from build123d import *

# Parameters (mm, degrees)
SKETCH_3_W          = 220
SKETCH_3_H          = 130
EXTRUDE_1_DEPTH     = 5
CUT_EXTRUDE_1_DEPTH = 6
SKETCH_3_4_W        = 220
SKETCH_3_4_H        = 13
EXTRUDE_2_DEPTH     = 15


with BuildPart() as part:
    # Sketch 3 → Extrude 1 (new body)
    with BuildSketch(Plane.XY):
        Rectangle(SKETCH_3_W, SKETCH_3_H)
    extrude(amount=EXTRUDE_1_DEPTH)

    # Sketch 3_3 → Cut-Extrude 1 (cut, through all)
    with BuildSketch(Plane.XY):
        Polygon((75.116731493, -11.546415335), (85.057854749, -5.672115229), (84.941123256, 5.874300106), (74.883268507, 11.546415335), (64.942145251, 5.672115229), (65.058876744, -5.874300106), align=None)
        Polygon((50.116731493, -11.546415335), (60.057854749, -5.672115229), (59.941123256, 5.874300106), (49.883268507, 11.546415335), (39.942145251, 5.672115229), (40.058876744, -5.874300106), align=None)
        Polygon((50.116731493, -41.546415335), (60.057854749, -35.672115229), (59.941123256, -24.125699894), (49.883268507, -18.453584665), (39.942145251, -24.327884771), (40.058876744, -35.874300106), align=None)
        Polygon((25.116731493, -41.546415335), (35.057854749, -35.672115229), (34.941123256, -24.125699894), (24.883268507, -18.453584665), (14.942145251, -24.327884771), (15.058876744, -35.874300106), align=None)
        Polygon((25.116731493, -11.546415335), (35.057854749, -5.672115229), (34.941123256, 5.874300106), (24.883268507, 11.546415335), (14.942145251, 5.672115229), (15.058876744, -5.874300106), align=None)
        Polygon((0.116731493, -41.546415335), (10.057854749, -35.672115229), (9.941123256, -24.125699894), (-0.116731493, -18.453584665), (-10.057854749, -24.327884771), (-9.941123256, -35.874300106), align=None)
        Polygon((-24.884546065, -41.546415335), (-14.943422809, -35.672115229), (-15.060154302, -24.125699894), (-25.118009051, -18.453584665), (-35.059132307, -24.327884771), (-34.942400814, -35.874300106), align=None)
        Polygon((-24.884546065, -11.546415335), (-14.943422809, -5.672115229), (-15.060154302, 5.874300106), (-25.118009051, 11.546415335), (-35.059132307, 5.672115229), (-34.942400814, -5.874300106), align=None)
        Polygon((0.116731493, -11.546415335), (10.057854749, -5.672115229), (9.941123256, 5.874300106), (-0.116731493, 11.546415335), (-10.057854749, 5.672115229), (-9.941123256, -5.874300106), align=None)
        Polygon((-49.885823623, -41.546415335), (-39.944700367, -35.672115229), (-40.06143186, -24.125699894), (-50.119286609, -18.453584665), (-60.060409866, -24.327884771), (-59.943678372, -35.874300106), align=None)
        Polygon((-49.885823623, -11.546415335), (-39.944700367, -5.672115229), (-40.06143186, 5.874300106), (-50.119286609, 11.546415335), (-60.060409866, 5.672115229), (-59.943678372, -5.874300106), align=None)
        Polygon((-74.887101181, -41.546415335), (-64.945977925, -35.672115229), (-65.062709418, -24.125699894), (-75.120564167, -18.453584665), (-85.061687424, -24.327884771), (-84.944955931, -35.874300106), align=None)
        Polygon((-74.887101181, 18.453584665), (-64.945977925, 24.327884771), (-65.062709418, 35.874300106), (-75.120564167, 41.546415335), (-85.061687424, 35.672115229), (-84.944955931, 24.125699894), align=None)
        Polygon((-49.885823623, 18.453584665), (-39.944700367, 24.327884771), (-40.06143186, 35.874300106), (-50.119286609, 41.546415335), (-60.060409866, 35.672115229), (-59.943678372, 24.125699894), align=None)
        Polygon((-24.884546065, 18.453584665), (-14.943422809, 24.327884771), (-15.060154302, 35.874300106), (-25.118009051, 41.546415335), (-35.059132307, 35.672115229), (-34.942400814, 24.125699894), align=None)
        Polygon((0.116731493, 18.453584665), (10.057854749, 24.327884771), (9.941123256, 35.874300106), (-0.116731493, 41.546415335), (-10.057854749, 35.672115229), (-9.941123256, 24.125699894), align=None)
        Polygon((25.116731493, 18.453584665), (35.057854749, 24.327884771), (34.941123256, 35.874300106), (24.883268507, 41.546415335), (14.942145251, 35.672115229), (15.058876744, 24.125699894), align=None)
        Polygon((50.116731493, 18.453584665), (60.057854749, 24.327884771), (59.941123256, 35.874300106), (49.883268507, 41.546415335), (39.942145251, 35.672115229), (40.058876744, 24.125699894), align=None)
        Polygon((75.116731493, 18.453584665), (85.057854749, 24.327884771), (84.941123256, 35.874300106), (74.883268507, 41.546415335), (64.942145251, 35.672115229), (65.058876744, 24.125699894), align=None)
        Polygon((85.057854749, -35.672115229), (84.941123256, -24.125699894), (74.883268507, -18.453584665), (64.942145251, -24.327884771), (65.058876744, -35.874300106), (75.116731493, -41.546415335), align=None)
        Polygon((-74.887101181, -11.546415335), (-64.945977925, -5.672115229), (-65.062709418, 5.874300106), (-75.120564167, 11.546415335), (-85.061687424, 5.672115229), (-84.944955931, -5.874300106), align=None)
    extrude(amount=CUT_EXTRUDE_1_DEPTH, mode=Mode.SUBTRACT)

    # Sketch 3_4 → Extrude 2 (add)
    with BuildSketch(Plane.XY):
        with Locations((0, 58.5)):
            Rectangle(SKETCH_3_4_W, SKETCH_3_4_H)
        with Locations((0, -58.5)):
            Rectangle(SKETCH_3_4_W, SKETCH_3_4_H)
    extrude(amount=EXTRUDE_2_DEPTH)


solid = part.part
Build history of the part. All positions in model axes, mm. Coordinates: 2 decimals unless noted, no trailing zeros. Write each loop counter-clockwise with the first axis right and the second up, starting at its lowest first coordinate (ties: lowest second). Pieces come first, ordered by that corner, then holes.
(1) Drill centre lines: line 1 (Y direction, x = 31, z = 13.25); line 2 (Y direction, x = 8, z = 1.5); line 3 (Z direction, x = -15, y = 22.5). Where is each one in solid material? Low to high.
(2) Cut at D-D on x = 19. List the corners of the cut face in (y, z).
(3) Cut at B-B on y = -22. State how many separate pieces and enclosed holes the cut face has, and give its area (3 significant figures).
(4) Mould opens along X. For faces 1 (the flat face through (-29.984, -38.671, 2.465)), 2 (the flat face through (4.98, -21.33, 2.46)) say: pulls with the +X half, pulls with the -X half, needs draft (parallel to the pull), parting line crosses it, or undercut.
(5) Cut at C-C on x = -90.5. List the corners of the cut face in (y, z), and give its area (3 significant figures).
(6) Pin check, flat tips, straight feed: pin 1 Ø6 at (y, z) = (-48.5, 6.5) entering from +X; pin 2 Ø10 at (x, y) = (49, 19) entering from +Z. Stop position of each tip, or through.
(7) Cut at A-A on z = 8.5. List the corners of the cut face in (x, y), and give its area (3 significant figures).
Working result:
1. line 1: y = -65 to -52, 52 to 65
1. line 2: y = -65 to -36.89, -23.03 to -6.89, 6.97 to 23.11, 36.97 to 65
1. line 3: z = 0 to 5
2. outline: (-65, 0) - (-38.1, 0) - (-38.1, 5) - (-52, 5) - (-52, 15) - (-65, 15) - close; (-21.93, 0) - (-8.1, 0) - (-8.1, 5) - (-21.93, 5) - close; (8.07, 0) - (21.9, 0) - (21.9, 5) - (8.07, 5) - close; (38.07, 0) - (65, 0) - (65, 15) - (52, 15) - (52, 5) - (38.07, 5) - close
3. separate pieces: 8
3. enclosed holes: 0
3. area: 670 mm2
4. face 1: undercut
4. face 2: undercut
5. outline: (-65, 0) - (65, 0) - (65, 15) - (52, 15) - (52, 5) - (-52, 5) - (-52, 15) - (-65, 15) - close
5. area: 910 mm2
6. pin 1: stops at x = 110
6. pin 2: stops at z = 5
7. outline: (-110, -65) - (110, -65) - (110, -52) - (-110, -52) - close; (-110, 52) - (110, 52) - (110, 65) - (-110, 65) - close
7. area: 5,720 mm2
